```python
from build123d import *

# Parameters (mm, degrees)
F1_R      = 4.85
F2_DEPTH  = 9.5
F6_R      = 2.5
F7_DEPTH  = 5
F8_R      = 2.3817700771
F9_DEPTH  = 2
F10_DEPTH = 1
F11_R     = 1.6629928967
F12_DEPTH = 10
F14_DEPTH = 13
F17_DEPTH = 2
F19_DEPTH = 2
F20_DEPTH = 2


with BuildPart() as f2:
    # F1 (on offset) → F2 (new body)
    with BuildSketch(Plane.XY.offset(-10)):
        Circle(F1_R)
    extrude(amount=-F2_DEPTH)

    # F3 (on Front) → F4 (revolve)
    with BuildSketch(Plane.XZ):
        with BuildLine():
            add(Edge.make_bspline(
                [(0, -9.970930405), (-1.3505217005, -10.321882545), (-4.7101037613, -11.3997414842), (-14.4883586925, 0.5183248415), (-9.7463505302, 10.1236115349), (-6.2063955702, 22.3837215453), (0, 21.5697698295)],
                knots=[0, 0, 0, 0, 0.1602983763, 0.4390878008, 0.7014553095, 1, 1, 1, 1], degree=3))
            Line((0, -9.970930405), (0, 21.5697698295))
        make_face()
    revolve(axis=Axis((0, 0, 5.7994197123), (0, 0, -1)))

    # F6 (on offset) → F7 (cut)
    with BuildSketch(Plane.XZ.offset(9)):
        with Locations((0, 7.3255817406)):
            Circle(F6_R)
    extrude(amount=F7_DEPTH, mode=Mode.SUBTRACT)

    # F8 (on offset) → F9 (join)
    with BuildSketch(Plane.XZ.offset(9)):
        with Locations((-2.5436044671, 12.0058143511)):
            Circle(F8_R)
        with Locations((2.5436044671, 12.0058143511)):
            Circle(F8_R)
    extrude(amount=F9_DEPTH)

    # F8 (on offset) → F10 (join)
    with BuildSketch(Plane.XZ.offset(9)):
        with Locations((-2.5436044671, 12.0058143511)):
            Circle(F8_R)
        with Locations((2.5436044671, 12.0058143511)):
            Circle(F8_R)
    extrude(amount=-F10_DEPTH)

    # F11 (on offset) → F12 (cut)
    with BuildSketch(Plane.XZ.offset(9)):
        with Locations((-2.5083974469, 11.8470387533)):
            Circle(F11_R)
        with Locations((2.5083974469, 11.8470387533)):
            Circle(F11_R)
    extrude(amount=F12_DEPTH, mode=Mode.SUBTRACT)

    # F13 (on Front) → F14 (cut)
    with BuildSketch(Plane.XZ):
        Polygon((8.6482558399, 3.2558140811), (-8.6482558399, 3.2558140811), (-9.2587219551, 3.2558140811), (-9.4622112811, 0), (-6.6133709624, -5.0872093998), (0, -7.7325585298), (6.6133709624, -5.0872093998), (9.4622112811, 0), (9.2587219551, 3.2558140811), align=None)
    extrude(amount=F14_DEPTH, mode=Mode.SUBTRACT)

    # F16 (on offset) → F17 (join)
    with BuildSketch(Plane.XZ.offset(12)):
        Polygon((0, 3.343462944), (-4.4047655538, 3.343462944), (-4.4047655538, 1.5467801131), (-3.6280222703, 0), (0, -1.0199095123), align=None)
        Polygon((4.4047655538, 3.343462944), (0, 3.343462944), (0, -1.0199095123), (3.6280222703, 0), (4.4047655538, 1.5467801131), align=None)
    extrude(amount=-F17_DEPTH)

    # F18 (on Front) → F19 (join)
    with BuildSketch(Plane.XZ):
        Polygon((-2.7080250438, 25.259565562), (-1.1835845653, 23.6207917333), (-0.650030619, 22.1725739539), (-0.6881413865, 20.9149103612), (-0.3440706932, 20.9530210122), (-0.3440706932, 23.2877233856), (-0.5356975016, 23.8875690848), (-1.9839156885, 25.412010029), (-5.528239999, 28.3084474504), (-5.528239999, 27.8624672941), align=None)
        Polygon((-0.3440706932, 23.2877233856), (-0.3440706932, 20.9530210122), (0, 20.9911316633), (0, 22.2106855363), align=None)
        Polygon((0, 22.2106855363), (0, 20.9911316633), (0.4551889142, 20.8767987788), (0.4551889142, 23.3921259642), (0.9125209763, 24.0781251341), (2.1320732776, 25.412010029), (4.7409896982, 27.4502248463), (4.5785000548, 28.0425772071), (2.4750723969, 26.3647846878), (0.9887429187, 25.1071210951), (0, 23.7351246178), align=None)
        Polygon((-0.3440706932, 25.259565562), (-0.3440706932, 23.2877233856), (0, 22.2106855363), (0, 23.7351246178), (0, 25.2214539796), (-0.3451424418, 27.7748927474), (-1.4884728007, 30.6332167238), (-1.7171388026, 30.213996768), (-0.7262525614, 27.0507819951), align=None)
    extrude(amount=F19_DEPTH)

    # F18 (on Front) → F20 (join)
    with BuildSketch(Plane.XZ):
        Polygon((-2.7080250438, 25.259565562), (-1.1835845653, 23.6207917333), (-0.650030619, 22.1725739539), (-0.6881413865, 20.9149103612), (-0.3440706932, 20.9530210122), (-0.3440706932, 23.2877233856), (-0.5356975016, 23.8875690848), (-1.9839156885, 25.412010029), (-5.528239999, 28.3084474504), (-5.528239999, 27.8624672941), align=None)
        Polygon((-0.3440706932, 23.2877233856), (-0.3440706932, 20.9530210122), (0, 20.9911316633), (0, 22.2106855363), align=None)
        Polygon((0, 22.2106855363), (0, 20.9911316633), (0.4551889142, 20.8767987788), (0.4551889142, 23.3921259642), (0.9125209763, 24.0781251341), (2.1320732776, 25.412010029), (4.7409896982, 27.4502248463), (4.5785000548, 28.0425772071), (2.4750723969, 26.3647846878), (0.9887429187, 25.1071210951), (0, 23.7351246178), align=None)
        Polygon((-0.3440706932, 25.259565562), (-0.3440706932, 23.2877233856), (0, 22.2106855363), (0, 23.7351246178), (0, 25.2214539796), (-0.3451424418, 27.7748927474), (-1.4884728007, 30.6332167238), (-1.7171388026, 30.213996768), (-0.7262525614, 27.0507819951), align=None)
    extrude(amount=-F20_DEPTH)


solid = f2.part
```
Source: CAD feature listing. Evaluate the final solid. Frame: model axes, mm. A direction names the side the tool comes from. Give positions to 0.01 mm unless a question says otherwise; leave off trailing zeros. Write each loop counter-clockwise with the first axis right and the second up, starting at its lowest first coordinate (ties: lowest second). Pieces come first, ordered by that corner, then holes. Notation, with made-up numbers: (75, 48) - (126, 48) arc R29 cw to (126, 87) - close; hole circle Ø4 at (-8.75, 45). An arc over 180 degrees is marked (long way). One line per item, written item: value. Start each with the question number.
Q1. Set-up query: faces 4 (the face through (3.42, -0.03, 26.42)), 5 (the face through (3.26, -3.78, -6.43)), 6 (the face through (4.626, 1.457, -14.683)), 7 (the face through (-1.839, -11.014, -0.503)), 8 (the face through (-4, 2, -10)). Return all of +Z, -Z, +X, -X, +Y, -Y with unobstructed straight access to the full face (end or side cutting, diameter ignored); none if empty.
Q2. Draft query along Z for faces 1 (the face through (-3.73, -0.03, 26.84)), 2 (the face through (1.789, -11.014, -0.517)), 3 (the face through (-4.14, -0.03, 26.58)). Return one class per face: +Z half, -Z half, draft (parallel to the pull), parting line (faces both ways), or undercut.
Q3. Material intervals for probe 1 along Z at (x, y) = (3.5, -1.75); probe 2 along X at (y, z) = (-10.5, 12.5); probe 3 along X at (y, z) = (-1.25, 22), sorted ascending. Write a range as from..to.
Q4. First-contact query: pin 1 Ø1.4 at (y, z) = (-11, 2.5) entering from +X; pin 2 Ø5 at (y, z) = (5.5, 4.5) entering from -X; pin 3 Ø3 at (x, z) = (2.51, 11.85) entering from -Y; pin 4 Ø6 at (x, z) = (-2.5, 5) entering from -Y. Flat tips, straight axial feed; report the tip coordinate or a pass-through.
Q5. Section query A-A, the plane z = -15. Return the cut outline in (x, y).
Answer:
1. face 4: +X, +Y, -Y
1. face 5: -Y
1. face 6: -Z
1. face 7: -Z, -X, -Y
1. face 8: none
2. face 1: +Z half
2. face 2: -Z half
2. face 3: undercut
3. probe 1: z = -19.5..-6.33, 3.26..20.94, 26.48..27.18
3. probe 2: x = -4.87..-4.04, -0.98..-0.21, 0.21..0.98, 4.04..4.87
3. probe 3: x = -0.66..0.46
4. pin 1: stops at x = 4.4
4. pin 2: stops at x = -11.75
4. pin 3: stops at y = -9
4. pin 4: stops at y = -12.2
5. outline: circle Ø9.7 at (0, 0)
